Design review of the part built by this model. Coordinates are the model's own, in mm. A direction names the side the tool comes from. Coordinates: 2 decimals unless noted, no trailing zeros. Order: outer loops, then holes, each group sorted by start corner. A loop starts at its lowest first (then second) coordinate and runs counter-clockwise, first axis right, second up.
from build123d import *

# Parameters (mm, degrees)
SKETCH1_W         = 1219.2
SKETCH1_H         = 1219.2
EXTRUDE1_DEPTH    = 25.4
FILLET1_R         = 25.4
EXTRUDE2_DEPTH    = 889
SKETCH3_W         = 6.35
SKETCH3_H         = 1066.8
EXTRUDE3_DEPTH    = 76.2
CIRPATTERN1_COUNT = 4


with BuildPart() as part:
    # Sketch1 → Extrude1 (new body)
    with BuildSketch(Plane(origin=(0, 0, 0), x_dir=(1, 0, 0), z_dir=(0, 1, 0))):
        Rectangle(SKETCH1_W, SKETCH1_H)
    extrude(amount=-EXTRUDE1_DEPTH)

    # Fillet1
    fillet1_edges = [part.edges().sort_by_distance(p)[0] for p in [
        (-609.6, -12.7, -609.6),
        (609.6, -12.7, -609.6),
        (609.6, -12.7, 609.6),
        (-609.6, -12.7, 609.6),
    ]]
    fillet(fillet1_edges, radius=FILLET1_R)

    # Sketch2 → Extrude2 (add)
    with BuildSketch(Plane.XZ.offset(25.4)):
        with BuildLine():
            Line((-469.9, 571.5), (-469.9, 565.15))
            Line((-469.9, 565.15), (-533.4, 565.15))
            ThreePointArc((-533.4, 565.15), (-555.850640303, 555.850640303), (-565.15, 533.4))
            Line((-565.15, 533.4), (-565.15, 469.9))
            Line((-565.15, 469.9), (-571.5, 469.9))
            Line((-571.5, 469.9), (-571.5, 533.4))
            ThreePointArc((-571.5, 533.4), (-560.340768363, 560.340768363), (-533.4, 571.5))
            Line((-533.4, 571.5), (-469.9, 571.5))
        make_face()
    extrude2 = extrude(amount=EXTRUDE2_DEPTH)

    # Sketch3 → Extrude3 (add)
    with BuildSketch(Plane.XZ.offset(25.4)):
        with Locations((-561.975, 0)):
            Rectangle(SKETCH3_W, SKETCH3_H)
    extrude3 = extrude(amount=EXTRUDE3_DEPTH)

    # CirPattern1: Extrude2, Extrude3 ×4 about axis
    cirpattern1_axis = Axis((0, 0, 0), (0, 1, 0))
    add([extrude2.rotate(cirpattern1_axis, i * 360 / CIRPATTERN1_COUNT) for i in range(1, CIRPATTERN1_COUNT)])
    add([extrude3.rotate(cirpattern1_axis, i * 360 / CIRPATTERN1_COUNT) for i in range(1, CIRPATTERN1_COUNT)])


solid = part.part
1. Add section A-A (y = -314.5). State how many separate pieces and enclosed holes the cut face has, and give its area (3 significant figures).
2. Insertion check: pin 1 (2 mm diameter, centred on x = -15.5, z = 218, fed in from +Y); pin 2 (1.9 mm diameter, centred on x = -561.5, z = -129, fed in from -Y); pin 3 (19 mm diameter, centred on x = 504.5, y = -262, fed in from +Z); pin 4 (7 mm diameter, centred on y = -690.5, z = -568.5, fed in from +X) (3 decimals). Each pin has a flat end and moves straight along its axis. Give the tip position at first contact, or say it passes through.
3. Mouldability with a two-part tool opening along X and no side actions: class faces 1 (the flat face through (-502, -502, -565.15)), 2 (the cylindrical face through (560.04, -463.68, 560.64)), 3 (the flat face through (502, -464, -571.5)), 4 (the flat face through (-7, -63, 565.15)) as pulls with the +X half, pulls with the -X half, needs draft (parallel to the pull), parting line crosses it, or undercut.
4. To check wall thickness, follow line 1 (Z direction, x = 391, y = -87.5); line 2 (X direction, y = -585, z = -471). State the ranges of each line that lie inside material, in increasing order.
5. Add section B-B (z = -406.5). Give the boundary of the cut face in (x, y).
6. Add section C-C (x = 135). Give the boundary of the cut face in (y, z).
7. For faces 5 (the flat face through (-571.5, -464, -502)), 6 (the cylindrical face through (-560.04, -463.68, -560.64)), 7 (the flat face through (558.8, -63, 7)), 8 (the flat face through (565.15, -63, 7)), 9 (the flat face through (501, -464, 571.5)), list the 3-axis set-ups (+Z, -Z, +X, -X, +Y, -Y) from which the entire face can be reached by the end or side of a thin tool; tool diameter is ignored.
Solution:
1. separate pieces: 4
1. enclosed holes: 0
1. area: 4,620 mm2
2. pin 1: stops at y = 0
2. pin 2: stops at y = -101.6
2. pin 3: stops at z = 571.5
2. pin 4: stops at x = 554.685
3. face 1: undercut
3. face 2: pulls with the +X half
3. face 3: needs draft
3. face 4: undercut
4. line 1: z = -565.15 to -558.8, 558.8 to 565.15
4. line 2: x = -571.5 to -565.15, 565.15 to 571.5
5. outline: (-609.6, -25.4) - (-565.15, -25.4) - (-565.15, -101.6) - (-558.8, -101.6) - (-558.8, -25.4) - (558.8, -25.4) - (558.8, -101.6) - (565.15, -101.6) - (565.15, -25.4) - (609.6, -25.4) - (609.6, 0) - (-609.6, 0) - close
6. outline: (-101.6, -565.15) - (-25.4, -565.15) - (-25.4, -609.6) - (0, -609.6) - (0, 609.6) - (-25.4, 609.6) - (-25.4, 565.15) - (-101.6, 565.15) - (-101.6, 558.8) - (-25.4, 558.8) - (-25.4, -558.8) - (-101.6, -558.8) - close
7. face 5: +Z, -Z, -X, -Y
7. face 6: -Z, -X, -Y
7. face 7: -Y
7. face 8: +X, -Y
7. face 9: +Z, +X, -X, -Y
